Autodesk Inventor part; units mm, degrees
ref_plane "YZ Plane" through (0, 0, 0) normal (1, 0, 0) x (0, 1, 0)
ref_plane "XZ Plane" through (0, 0, 0) normal (0, 1, 0) x (-1, 0, 0)
ref_plane "XY Plane" through (0, 0, 0) normal (0, 0, 1) x (1, 0, 0)
sketch "Sketch1" plane through (0, 0, 0) normal (0, 1, 0) x (-1, 0, 0)
  circle A0 centre (0, 0) radius 4.9
  circle A1 centre (0, 0) radius 3.1
  dimension "d0" = 9.8
  dimension "d1" = 6.2
extrude "Extrusion1" add sketch "Sketch1" along normal blind 6
sketch "Sketch2" plane through (0, 0, 0) normal (0, -1, 0) x (1, 0, 0)
  circle A0 centre (0, 0) radius 6
  circle A1 centre (0, 0) radius 4.9
  circle A2 centre (0, 0) radius 3.1
  dimension "d4" = 12
extrude "Extrusion2" add sketch "Sketch2" against normal blind 2 contours A0
fillet "Fillet1" radius 0.75 1 edges at (4.9, 6, 0)
properties part number "bøsning_beslag_3D" material "Brass, Soft Yellow"
CAD build for the part. Positions are in the model's coordinates, mm. A direction names the side the tool comes from. Round coordinates to 2 decimals unless told otherwise and drop trailing zeros. Order: outer loops, then holes, each group sorted by start corner. A loop starts at its lowest first (then second) coordinate and runs counter-clockwise, first axis right, second up.
Q1. Slice it at C-C (y = 2.3). Write the cut outline in (x, z).
Q2. Which spindle directions (+Z, -Z, +X, -X, +Y, -Y) get a long thin tool onto all of the face, cutting with end or side? Do faces 1 (the flat face through (3, 0, -3)), 2 (the flat face through (1, 2, -5)). Say none if no direction does.
Q3. Drop flat-ended pins along their axis: pin 1 (1.5 mm diameter, centred on x = 1, y = 2, fed in from +Z); pin 2 (3 mm diameter, centred on y = 5, z = -0.5, fed in from -X); pin 3 (1 mm diameter, centred on x = 3.5, y = 1.5, fed in from -Z). Give the stop position or say it passes through.
Q4. Slice it at D-D (y = 5.65). Write the cut outline in (x, z).
Q5. Slice it at B-B (x = 0). Write the cut outline in (y, z).
Q6. Slice it at A-A (z = 0). Write the cut outline in (x, y).
Q7. Wall check: L1, parallel to Z at x = 0, y = 1.85; L2, parallel to Z at x = 0, y = 2.5; L3, parallel to Y at x = -2.25, z = -5.25. Give the ranges that are in metal, low to high.
Q8. Two-plate mould, pull along Z, no slides. Class faces 3 (the flat face through (2, 6, -3)), 4 (the cylindrical face through (-1.43, 2.96, 2.75)), 5 (the cylindrical face through (-6, 1, 0)): pulls with the +Z half, pulls with the -Z half, needs draft (parallel to the pull), parting line crosses it, or undercut.
Results below:
1. outline: circle Ø9.8 at (0, 0); hole circle Ø6.2 at (0, 0)
2. face 1: +Z, -Z, +X, -X, -Y
2. face 2: +Y
3. pin 1: stops at z = 5.99
3. pin 2: stops at x = -4.9
3. pin 3: stops at z = -5.2
4. outline: circle Ø9.57 at (0, 0); hole circle Ø6.2 at (0, 0)
5. outline: (0, -6) - (2, -6) - (2, -4.9) - (5.25, -4.9) arc R0.75 ccw to (6, -4.15) - (6, -3.1) - (0, -3.1) - close; (0, 3.1) - (6, 3.1) - (6, 4.15) arc R0.75 ccw to (5.25, 4.9) - (2, 4.9) - (2, 6) - (0, 6) - close
6. outline: (-6, 0) - (-3.1, 0) - (-3.1, 6) - (-4.15, 6) arc R0.75 ccw to (-4.9, 5.25) - (-4.9, 2) - (-6, 2) - close; (3.1, 0) - (6, 0) - (6, 2) - (4.9, 2) - (4.9, 5.25) arc R0.75 ccw to (4.15, 6) - (3.1, 6) - close
7. L1: z = -6 to -3.1, 3.1 to 6
7. L2: z = -4.9 to -3.1, 3.1 to 4.9
7. L3: y = 0 to 2
8. face 3: needs draft
8. face 4: undercut
8. face 5: parting line crosses it
